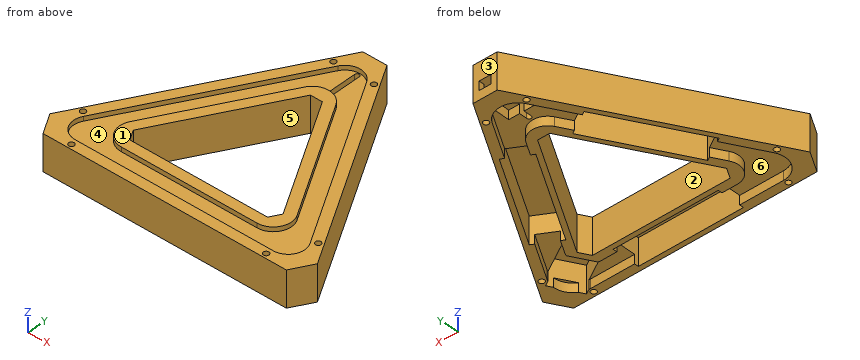
from build123d import *

# Parameters (mm, degrees)
PAD_DEPTH             = 24
POCKET_DEPTH          = 3
SKETCH002_W           = 70
SKETCH002_H           = 18.5
POCKET001_DEPTH       = 18
POLARPATTERN_COUNT    = 3
POCKET002_DEPTH       = 6
CHAMFER_SIZE          = 8
FILLET_R              = 13
FILLET001_R           = 11
CHAMFER001_SIZE       = 16.1
FILLET002_R           = 11
FILLET003_R           = 12
POCKET003_DEPTH       = 6
POCKET004_DEPTH       = 18
POCKET005_DEPTH       = 21.001
SKETCH012_R           = 1.85
POCKET011_DEPTH       = 498.049286
POLARPATTERN001_COUNT = 3


with BuildPart() as part:
    # Sketch → Pad (new body)
    with BuildSketch(Plane.XY):
        Polygon((0, 112.209492), (-97.17627, -56.104746), (97.17627, -56.104746), align=None)
        Polygon((0, 62.209492), (-53.875, -31.104746), (53.875, -31.104746), align=None, mode=Mode.SUBTRACT)
    extrude(amount=PAD_DEPTH)

    # Sketch001 (on Face8 of Pad) → Pocket (cut)
    with BuildSketch(Plane.XY.offset(24)):
        Polygon((0, 98.209492), (-85.051915, -49.104746), (85.051915, -49.104746), align=None)
        Polygon((0, 76.209492), (-65.999356, -38.104746), (65.999356, -38.104746), align=None, mode=Mode.SUBTRACT)
    extrude(amount=-POCKET_DEPTH, mode=Mode.SUBTRACT)

    # Sketch002 (on Face4 of Pocket) → Pocket001 (cut)
    with BuildSketch(Plane(origin=(0, 0, 0), x_dir=(1, 0, 0), z_dir=(0, 0, -1))):
        with Locations((0, 43.604746)):
            Rectangle(SKETCH002_W, SKETCH002_H)
    pocket001 = extrude(amount=-POCKET001_DEPTH, mode=Mode.SUBTRACT)

    # PolarPattern: Pocket001 ×3 about axis
    polarpattern_axis = Axis((0, 0, 0), (0, 0, -1))
    for i in range(1, POLARPATTERN_COUNT):
        add(pocket001.rotate(polarpattern_axis, i * 360 / POLARPATTERN_COUNT), mode=Mode.SUBTRACT)

    # Sketch003 (on Face4 of PolarPattern) → Pocket002 (cut)
    with BuildSketch(Plane(origin=(0, 0, 0), x_dir=(1, 0, 0), z_dir=(0, 0, -1))):
        Polygon((0, -100.209492), (86.783965, 50.104746), (-86.783965, 50.104746), align=None)
        Polygon((0, -74.209492), (64.267305, 37.104746), (-64.267305, 37.104746), align=None, mode=Mode.SUBTRACT)
    extrude(amount=-POCKET002_DEPTH, mode=Mode.SUBTRACT)

    # Chamfer
    chamfer_edges = [part.edges().sort_by_distance(p)[0] for p in [
        (-53.875, -31.104746, 12),
        (53.875, -31.104746, 12),
        (0, 62.209492, 12),
    ]]
    chamfer(chamfer_edges, length=CHAMFER_SIZE)

    # Fillet
    fillet_edges = [part.edges().sort_by_distance(p)[0] for p in [
        (0, 100.209492, 3),
        (-86.783965, -50.104746, 3),
        (86.783965, -50.104746, 3),
    ]]
    fillet(fillet_edges, radius=FILLET_R)

    # Fillet001
    fillet001_edges = [part.edges().sort_by_distance(p)[0] for p in [
        (0, 74.209492, 3),
        (64.267305, -37.104746, 3),
        (-64.267305, -37.104746, 3),
    ]]
    fillet(fillet001_edges, radius=FILLET001_R)

    # Chamfer001
    chamfer001_edges = [part.edges().sort_by_distance(p)[0] for p in [
        (97.17627, -56.104746, 12),
        (0, 112.209492, 12),
        (-97.17627, -56.104746, 12),
    ]]
    chamfer(chamfer001_edges, length=CHAMFER001_SIZE)

    # Fillet002
    fillet002_edges = [part.edges().sort_by_distance(p)[0] for p in [
        (0, 98.209492, 22.5),
        (-85.051915, -49.104746, 22.5),
        (85.051915, -49.104746, 22.5),
    ]]
    fillet(fillet002_edges, radius=FILLET002_R)

    # Fillet003
    fillet003_edges = [part.edges().sort_by_distance(p)[0] for p in [
        (65.999356, -38.104746, 22.5),
        (0, 76.209492, 22.5),
        (-65.999356, -38.104746, 22.5),
    ]]
    fillet(fillet003_edges, radius=FILLET003_R)

    # Sketch004 (on Face60 of Fillet003) → Pocket003 (cut)
    with BuildSketch(Plane(origin=(0, 0, 6), x_dir=(1, 0, 0), z_dir=(0, 0, -1))):
        Polygon((-8.75, -71.266483), (8.75, -71.266483), (8.75, -94.766483), (4, -94.766483), (4, -98.266483), (-4, -98.266483), (-4, -94.766483), (-8.75, -94.766483), align=None)
    extrude(amount=-POCKET003_DEPTH, mode=Mode.SUBTRACT)

    # Sketch005 (on Face29 of Pocket003) → Pocket004 (cut)
    with BuildSketch(Plane(origin=(0, 0, 0), x_dir=(1, 0, 0), z_dir=(0, 0, -1))):
        Polygon((46.171599, 38.954746), (68.688259, 51.954746), (79.338259, 33.508405), (56.821599, 20.508405), align=None)
    extrude(amount=-POCKET004_DEPTH, mode=Mode.SUBTRACT)

    # Sketch006 (on Face1 of Pocket004) → Pocket005 (cut, through all)
    with BuildSketch(Plane.XY.offset(21)):
        with BuildLine():
            ThreePointArc((1.5, 85.040452), (0, 86.540452), (-1.5, 85.040452))
            Line((-1.5, 85.040452), (-1.5, 66.040452))
            ThreePointArc((-1.5, 66.040452), (0, 64.540452), (1.5, 66.040452))
            Line((1.5, 85.040452), (1.5, 66.040452))
        make_face()
    extrude(amount=-POCKET005_DEPTH, mode=Mode.SUBTRACT)

    # Sketch012 → Pocket011 (cut, through all)
    with BuildSketch(Plane(origin=(0, 0, 0), x_dir=(1, 0, 0), z_dir=(0, 0, -1))):
        with Locations((-13.5, -82.703211)):
            Circle(SKETCH012_R)
        with Locations((13.5, -82.703211)):
            Circle(SKETCH012_R)
    pocket011 = extrude(amount=-POCKET011_DEPTH, mode=Mode.SUBTRACT)

    # PolarPattern001: Pocket011 ×3 about axis
    polarpattern001_axis = Axis((0, 0, 0), (0, 0, -1))
    for i in range(1, POLARPATTERN001_COUNT):
        add(pocket011.rotate(polarpattern001_axis, i * 360 / POLARPATTERN001_COUNT), mode=Mode.SUBTRACT)


solid = part.part
Can you work these out from the model? Positions are in its coordinate system, mm. Face numbers are marked on the shaded views. A direction names the side the tool comes from. Coordinates: 2 decimals unless noted, no trailing zeros. Write each loop counter-clockwise with the first axis right and the second up, starting at its lowest first coordinate (ties: lowest second). Pieces come first, ordered by that corner, then holes. Notation, with made-up numbers: (-32.5, 80) -> (6.5, 80) arc R16 ccw to (6.5, 85) -> close; hole circle Ø7 at (52.5, 35). An arc over 180 degrees is marked (long way). Write each question's results on one line, items separated by ' | '. Start each with the question number.
Q1. Imagine slicing it at C-C (z = 3.75). State how many separate pieces and enclosed holes the cut face has, then the cut area to 3 significant figures.
Q2. We'd pull the mould along Y, two halves only. Please class the marked faces 1, 2 and 3: +Y half, -Y half, draft (parallel to the pull), parting line (faces both ways), or undercut.
Q3. If I drill on probe 1 along Y at (x, z) = (-31, 10.5); probe 2 along X at (y, z) = (55, 2); probe 3 along Y at (x, z) = (-14, 9.25), over which ranges is the centre line in solid material (lowest first)?
Q4. Imagine slicing it at B-B (x = -19.5). Write out the boundary of the cut face in (y, z), then the cut area to 3 significant figures.
Q5. On a 3-axis mill with a long thin cutter (end or side, diameter ignored), from which of +Z, -Z, +X, -X, +Y, -Y can I reach the whole of each face in a straight line? I mean the marked faces 4, 5 and 6. Say none if no direction works.
Q6. Imagine slicing it at A-A (y = 53). Write out the boundary of the cut face in (x, z).
Q7. I'm going to push flat-ended pins straight in: pin 1 (1.8 mm diameter, centred on y = 81.5, z = 10, fed in from +X); pin 2 (6 mm diameter, centred on x = -35, y = 16.5, fed in from +Z); pin 3 (3.5 mm diameter, centred on x = 17, z = 22, fed in from +Y); pin 4 (7 mm diameter, centred on x = -16.5, z = 9.5, fed in from +Y). Where does each tip first touch, or does it pass through?
Taken from the geometry:
1) separate pieces: 2 | enclosed holes: 8 | area: 4,010 mm^2
2) face 1: draft | face 2: undercut | face 3: +Y half
3) probe 1: y = -56.1 to -52.85, -34.35 to -31.1, 8.52 to 15.02, 52.02 to 58.52 | probe 2: x = -33.03 to -29.28, -11.09 to -4.16, 4.16 to 11.09, 29.28 to 33.03 | probe 3: y = -56.1 to -52.85, -34.35 to -31.1, 37.96 to 44.46, 48.5 to 80.92, 84.48 to 87.96
4) outline: (-56.1, 0) -> (-52.85, 0) -> (-52.85, 18) -> (-34.35, 18) -> (-34.35, 0) -> (-31.1, 0) -> (-31.1, 24) -> (-38.1, 24) -> (-38.1, 21) -> (-49.1, 21) -> (-49.1, 24) -> (-56.1, 24) -> close; (28.43, 0) -> (34.93, 0) -> (34.93, 18) -> (51.67, 18) -> (51.67, 6) -> (66.43, 6) -> (66.43, 0) -> (78.43, 0) -> (78.43, 24) -> (64.43, 24) -> (64.43, 21) -> (42.43, 21) -> (42.43, 24) -> (28.43, 24) -> close | area: 978 mm^2
5) face 4: +Z | face 5: +Z, -Z | face 6: -Z
6) outline: (-34.18, 0) -> (-30.43, 0) -> (-30.43, 18) -> (-21.8, 18) -> (-21.8, 6) -> (-12.25, 6) -> (-12.25, 0) -> (-5.32, 0) -> (-5.32, 24) -> (-13.4, 24) -> (-13.4, 21) -> (-26.1, 21) -> (-26.1, 24) -> (-34.18, 24) -> close; (5.32, 0) -> (12.25, 0) -> (12.25, 6) -> (21.8, 6) -> (21.8, 18) -> (30.43, 18) -> (30.43, 0) -> (34.18, 0) -> (34.18, 24) -> (26.1, 24) -> (26.1, 21) -> (13.4, 21) -> (13.4, 24) -> (5.32, 24) -> close
7) pin 1: stops at x = 18.25 | pin 2: stops at z = 24 | pin 3: stops at y = 85.8 | pin 4: stops at y = 89.69
